```python
from build123d import *

# Parameters (mm, degrees)
IZIM1_R                     = 15
Y_KSEKLIK_EKSTR_ZYON1_DEPTH = 1
IZIM2_R                     = 11.118013459
Y_KSEKLIK_EKSTR_ZYON2_DEPTH = 15
IZIM3_R                     = 2
KES_EKSTR_ZYON1_DEPTH       = 38.810359459


with BuildPart() as part:
    # Çizim1 → Yükseklik-Ekstrüzyon1 (new body)
    with BuildSketch(Plane.XY):
        with Locations((-15.799728609, 0)):
            Circle(IZIM1_R)
    extrude(amount=Y_KSEKLIK_EKSTR_ZYON1_DEPTH)

    # Çizim2 → Yükseklik-Ekstrüzyon2 (add)
    with BuildSketch(Plane.XY.offset(1)):
        with Locations((-15.799728609, 0)):
            Circle(IZIM2_R)
    extrude(amount=Y_KSEKLIK_EKSTR_ZYON2_DEPTH)

    # Çizim3 → Kes-Ekstrüzyon1 (cut, through all)
    with BuildSketch(Plane.XY.offset(16)):
        with Locations((-15.799728609, 0)):
            Circle(IZIM3_R)
    extrude(amount=-KES_EKSTR_ZYON1_DEPTH, mode=Mode.SUBTRACT)


solid = part.part
```
Geometry check sheet. Reference: the model listing, model coordinates, mm. A direction names the side the tool comes from. Give positions to 0.01 mm unless a question says otherwise; leave off trailing zeros. Write each loop counter-clockwise with the first axis right and the second up, starting at its lowest first coordinate (ties: lowest second). Pieces come first, ordered by that corner, then holes.
1) Access from +Z, -Z, +X, -X, +Y, -Y to the whole of each face (thin tool, end or side, straight path). Record for faces 1 (the flat face through (-26, -5, 1)), 2 (the flat face through (-13, 0, 16)).
2) Section check C-C, the plane y = -5. Record the boundary of the cut face in (x, z), and give its area (3 significant figures).
3) Material ranges on L1, parallel to Z at x = -3.75, y = 5.5; L2, parallel to Y at x = -23.75, z = 2.25; L3, parallel to Y at x = -23.25, z = 7, recorded low to high.
4) Gauge pin test, flat ends, axial feed: pin 1 (5 mm diameter, centred on x = -9.5, z = 4.5, fed in from -Y); pin 2 (5 mm diameter, centred on x = -17.5, z = 5, fed in from -Y); pin 3 (6 mm diameter, centred on x = -22, z = 7, fed in from +Y). Record the tip position at first contact, or that the pin passes through.
5) Section check D-D, the plane z = 1.5. Record the boundary of the cut face in (x, y).
6) Section check B-B, the plane x = -16.25. Record the boundary of the cut face in (y, z), and give its area (3 significant figures).
7) Release check for a two-part mould opening along Y. For faces 3 (the flat face through (-13, 0, 0)), 4 (the cylindrical face through (-13.952, -0.766, 8.112)), 5 (the cylindrical face through (-26.907, 0.489, 8.395)) record: pulls with the +Y half, pulls with the -Y half, needs draft (parallel to the pull), parting line crosses it, or undercut.
8) Section check A-A, the plane y = 0. Record the boundary of the cut face in (x, z).
Computed:
1. face 1: +Z
1. face 2: +Z, +X, -X, +Y, -Y
2. outline: (-29.94, 0) - (-1.66, 0) - (-1.66, 1) - (-5.87, 1) - (-5.87, 16) - (-25.73, 16) - (-25.73, 1) - (-29.94, 1) - close
2. area: 326 mm2
3. L1: z = 0 to 1
3. L2: y = -7.77 to 7.77
3. L3: y = -8.25 to 8.25
4. pin 1: stops at y = -10.45
4. pin 2: stops at y = -11.12
4. pin 3: stops at y = 10.65
5. outline: circle Ø22.24 at (-15.8, 0); hole circle Ø4 at (-15.8, 0)
6. outline: (-14.99, 0) - (-1.95, 0) - (-1.95, 16) - (-11.11, 16) - (-11.11, 1) - (-14.99, 1) - close; (1.95, 0) - (14.99, 0) - (14.99, 1) - (11.11, 1) - (11.11, 16) - (1.95, 16) - close
6. area: 301 mm2
7. face 3: needs draft
7. face 4: undercut
7. face 5: parting line crosses it
8. outline: (-30.8, 0) - (-17.8, 0) - (-17.8, 16) - (-26.92, 16) - (-26.92, 1) - (-30.8, 1) - close; (-13.8, 0) - (-0.8, 0) - (-0.8, 1) - (-4.68, 1) - (-4.68, 16) - (-13.8, 16) - close
